from build123d import *

# Parameters (mm, degrees)
F1_DEPTH = 352.425
F2_W     = 22.225
F2_H     = 3.96875
F3_DEPTH = 25.4
F5_DEPTH = 38.1


with BuildPart() as f1:
    # F0 (on Front) → F1 (new body)
    with BuildSketch(Plane.XZ):
        Polygon((-18.553972, 20.450408), (-21.728972, 20.450408), (-21.728972, -17.649592), (16.371028, -17.649592), (16.371028, -14.474592), (-18.553972, -14.474592), align=None)
    extrude(amount=F1_DEPTH)

    # F2 (on face) → F3 (cut)
    with BuildSketch(Plane.YZ.offset(-18.553972)):
        with Locations((-11.1125, 18.466033)):
            Rectangle(F2_W, F2_H)
    extrude(amount=-F3_DEPTH, mode=Mode.SUBTRACT)

    # F4 (on face) → F5 (cut)
    with BuildSketch(Plane(origin=(0, 0, -17.649592), x_dir=(1, 0, 0), z_dir=(0, 0, -1))):
        Polygon((16.371028, 352.425), (-21.728972, 352.425), (16.371028, 314.325), align=None)
    extrude(amount=-F5_DEPTH, mode=Mode.SUBTRACT)


solid = f1.part
Verification items for the finished model (mm, model axes). A direction names the side the tool comes from. Give positions to 0.01 mm unless a question says otherwise; leave off trailing zeros. Write each loop counter-clockwise with the first axis right and the second up, starting at its lowest first coordinate (ties: lowest second). Pieces come first, ordered by that corner, then holes.
(1) Material ranges on line 1 (X direction, y = -258.5, z = 17.5); line 2 (Z direction, x = 5, y = -132.5); line 3 (Y direction, x = -5, z = -15), recorded low to high.
(2) Cross-section at A-A (y = -71). Enter the section's corners in (x, z), plus the area to 3 significant figures.
(3) Gauge pin test, flat ends, axial feed: pin 1 (4 mm diameter, centred on x = -17.5, z = 15.5, fed in from -Y); pin 2 (12 mm diameter, centred on x = -7, y = -178, fed in from +Z); pin 3 (1 mm diameter, centred on x = -19.5, z = 18, fed in from +Y) (3 decimals); pin 4 (8 mm diameter, centred on x = 5, z = -7.5, fed in from -Y). Record the tip position at first contact, or that the pin passes through.
(4) Cross-section at C-C (x = 4.5). Enter the section's corners in (y, z).
(5) Cross-section at B-B (z = -7.5). Enter the section's corners in (x, y) (3 decimals).
(6) Access from +Z, -Z, +X, -X, +Y, -Y to the whole of each face (thin tool, end or side, straight path). Record for faces 1 (the face through (-21.729, -174, 2)), 2 (the face through (-18.554, -172, 3)).
Worked out:
1. line 1: x = -21.73 to -18.55
1. line 2: z = -17.65 to -14.47
1. line 3: y = -335.7 to 0
2. outline: (-21.73, -17.65) - (16.37, -17.65) - (16.37, -14.47) - (-18.55, -14.47) - (-18.55, 20.45) - (-21.73, 20.45) - close
2. area: 232 mm2
3. pin 1: stops at y = -350.2
3. pin 2: stops at z = -14.47
3. pin 3: stops at y = -22.225
3. pin 4: passes through
4. outline: (-326.2, -17.65) - (0, -17.65) - (0, -14.47) - (-326.2, -14.47) - close
5. outline: (-21.729, -352.425) - (-18.554, -349.25) - (-18.554, 0) - (-21.729, 0) - close
6. face 1: +Z, -Z, -X, +Y, -Y
6. face 2: +Z, +X, +Y, -Y
